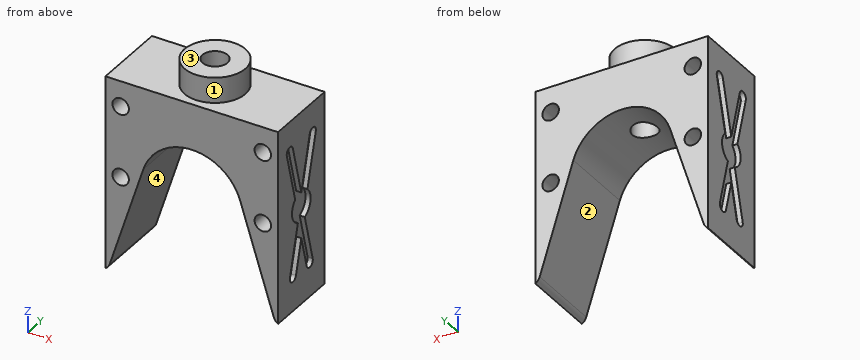
Autodesk Inventor part; units mm, degrees
ref_plane "Work Plane1" through (-17, 0, 0) normal (1, 0, 0) x (0, 1, 0)
ref_plane "XZ Plane" through (0, 0, 0) normal (0, 1, 0) x (-1, 0, 0)
ref_plane "XY Plane" through (0, 0, 0) normal (0, 0, 1) x (1, 0, 0)
sketch "Sketch1" plane through (0, 0, 0) normal (0, 1, 0) x (-1, 0, 0)
  line L0 (0, 0) -> (34, 0)
  line L1 (34, 0) -> (34, -38)
  line L2 (34, -38) -> (0, -38)
  line L3 (0, -38) -> (0, 0)
  point P0 (17, -38)
  dimension "d0" = 34
  dimension "d1" = 38
extrude "Extrusion1" add sketch "Sketch1" along normal blind 15
sketch "Sketch2" plane through (0, 15, 0) normal (0, 1, 0) x (1, 0, 0)
  arc A0 (-26.5342, 15.9835) -> (-7.4658, 15.9835) centre (-17, 19) ccw
  line L0 (-26.5342, 15.9835) -> (-33.5, 38)
  line L1 (0, 38) -> (-34, 38)
  line L2 (-7.4658, 15.9835) -> (-0.5, 38)
  point P0 (0, 0)
  point P1 (-17, 38)
  dimension "d4" = 16.5
  dimension "d5" = 16.5
  dimension "d6" = 10
  dimension "d7" = 19
extrude "Extrusion2" cut sketch "Sketch2" against normal up to surface (15 mm away)
fillet "Fillet1" radius 2 2 edges at (-0.5, 7.5, -38) (-33.5, 7.5, -38)
sketch "Sketch3" plane through (0, 15, 0) normal (0, 1, 0) x (1, 0, 0)
  line L0 (-34, 0) -> (0, 0)
  point P0 (-3, 19)
  point P1 (-31, 19)
  point P2 (-17, 0)
  point P3 (-17, 0)
  point P4 (-34, 38)
  dimension "d19" = 14
  dimension "d20" = 14
  dimension "d59" = 19
hole "Hole1" at (-3, 15, -19) at (-31, 15, -19) direction (0, -1, 0) diameter 3.242 depth 15
sketch "Sketch4" plane through (0, 15, 0) normal (0, 1, 0) x (1, 0, 0)
  line L0 (-34, 0) -> (0, 0)
  point P0 (-31, 5)
  point P1 (-3, 5)
  point P2 (-17, 0)
  point P3 (-17, 0)
  dimension "d28" = 14
  dimension "d29" = 14
  dimension "d30" = 5
hole "Hole2" at (-31, 15, -5) at (-3, 15, -5) direction (0, -1, 0) diameter 3.242 depth 15
sketch "Sketch5" plane through (-34, 0, 0) normal (0, 0, 1) x (1, 0, 0)
  circle A0 centre (17, 7.5) radius 6
  line L0 (0, 0) -> (34, 0)
  line L1 (0, 0) -> (0, 15)
  point P0 (17, 0)
  point P1 (0, 7.5)
  dimension "d31" = 12
extrude "Extrusion3" add sketch "Sketch5" along normal blind 5
sketch "Sketch6" plane through (-17, 7.5, 5) normal (0, 0, 1) x (1, 0, 0)
  circle A0 centre (0, 0) radius 6
  point P0 (17, -7.5)
hole "Hole3" at (-17, 7.5, 5) direction (0, 0, -1) diameter 4.917 depth 15
sketch "Sketch7" plane through (-34, 0, -38) normal (-1, 0, 0) x (0, 0, 1)
  line L0 (16.5986, 8.6063) -> (7.046, 11.1659)
  arc A0 (7.046, 11.1659) -> (6.5283, 9.2341) centre (6.7872, 10.2) ccw
  line L1 (6.5283, 9.2341) -> (13, 7.5)
  line L2 (13, 7.5) -> (6.5283, 5.7659)
  arc A1 (6.5283, 5.7659) -> (7.046, 3.8341) centre (6.7872, 4.8) ccw
  line L3 (7.046, 3.8341) -> (16.5986, 6.3937)
  line L4 (21.653, 9.4662) -> (31.7283, 12.1659)
  arc A2 (32.246, 10.2341) -> (31.7283, 12.1659) centre (31.9872, 11.2) ccw
  line L5 (32.246, 10.2341) -> (22.0423, 7.5)
  line L6 (22.0423, 7.5) -> (32.246, 4.7659)
  arc A3 (31.7283, 2.8341) -> (32.246, 4.7659) centre (31.9872, 3.8) ccw
  line L7 (31.7283, 2.8341) -> (21.653, 5.5338)
  line L8 (0, 0) -> (0, 15)
  line L9 (0, 7.5) -> (36.5337, 7.5) construction
  arc A4 (16.5986, 6.3937) -> (21.653, 5.5338) centre (19.3872, 7.5) ccw
  arc A5 (21.653, 9.4662) -> (16.5986, 8.6063) centre (19.3872, 7.5) ccw
  line L10 (0, 15) -> (38, 15)
  point P0 (38, 0)
  point P1 (11.8223, 5.1139)
  dimension "d42" = 2
  dimension "d43" = 2
  dimension "d44" = 2
  dimension "d45" = 2
  dimension "d46" = 12.6
  dimension "d47" = 12.6
  dimension "d48" = 26
  dimension "d49" = 26
  dimension "d50" = 30
  dimension "d51" = 30
  dimension "d52" = 3.8
  dimension "d53" = 3
  dimension "d54" = 3
  dimension "d55" = 13
extrude "Extrusion4" cut sketch "Sketch7" against normal blind 1
ref_plane "Work Plane1" through (-17, 0, 0) normal (1, 0, 0) x (0, 1, 0)
mirror "Mirror1" about plane through (-17, 0, 0) normal (1, 0, 0) of "Extrusion4"
equation "\"d5\" = d4"
equation "\"d12\" = d20"
equation "\"d44\" = d43"
equation "\"d47\" = d46"
equation "\"d54\" = d53"
properties part number "2023"
The listing builds one solid part. Answer for the finished solid, in the listing's coordinates (mm). Face numbers are marked on the shaded views. Coordinates: 2 decimals unless noted, no trailing zeros. Write each loop counter-clockwise with the first axis right and the second up, starting at its lowest first coordinate (ties: lowest second). Pieces come first, ordered by that corner, then holes. Notation, with made-up numbers: M 55,84.5 L 59,84.5 A30 ccw 59,115.5 Z; hole C -11.5,-22 d8. An arc over 180 degrees is marked long. Use a Markdown table: item, result. Add a question column.
1. Section B-B (z = -2) is taken. Give the vertices of the cut face in (x, y).
2. Section D-D (z = -19) is taken. Give the vertices of the cut face in (x, y).
3. Given P1, Ø1.9, axis at x = -31, z = -5, coming from the +Y side, flat-ended and moving along its own axis, determine where the tip first touches the part or whether it passes through.
4. Straight lines are drawn through the part: line 1 along X through (y, z) = (5.5, -5); line 2 along X through (y, z) = (7.5, -5); line 3 along X through (y, z) = (11.5, -11). For each, find the intervals that lie inside material, in ascending order. Write a range as [from, to].
5. Section C-C (x = -3) is taken. Give the vertices of the cut face in (y, z), plus the area to 3 significant figures.
6. Section A-A (x = -17) is taken. Give the vertices of the cut face in (y, z), plus the area to 3 significant figures.
7. For a pull along X with two mould halves and no side action, classify the marked faces 1, 2, 3 and 4 as +X half, -X half, draft (parallel to the pull), parting line (faces both ways), or undercut.
Data:
| question | item | result |
|---|---|---|
| 1 | outline | M -34,0 L 0,0 L 0,15 L -34,15 Z; hole C -17,7.5 d4.92 |
| 2 | outline | M -34,0 L -32.62,0 L -32.62,15 L -34,15 L -34,10.47 L -33,10.47 L -33,4.53 L -34,4.53 Z; M -29.38,0 L -27.49,0 L -27.49,15 L -29.38,15 Z; M -6.51,0 L -4.62,0 L -4.62,15 L -6.51,15 Z; M -1.38,0 L 0,0 L 0,4.53 L -1,4.53 L -1,10.47 L 0,10.47 L 0,15 L -1.38,15 Z |
| 3 | P1 | passes through |
| 4 | line 1 | x = [-34, -32.62], [-29.38, -18.43], [-15.57, -4.62], [-1.38, 0] |
| 4 | line 2 | x = [-34, -32.62], [-29.38, -19.46], [-14.54, -4.62], [-1.38, 0] |
| 4 | line 3 | x = [-34, -23], [-11, 0] |
| 5 | outline | M 0,-30.1 L 15,-30.1 L 15,-20.62 L 0,-20.62 Z; M 0,-17.38 L 15,-17.38 L 15,-6.62 L 0,-6.62 Z; M 0,-3.38 L 15,-3.38 L 15,0 L 0,0 Z |
| 5 | area | 354 mm2 |
| 6 | outline | M 0,-9 L 5.04,-9 L 5.04,5 L 1.5,5 L 1.5,0 L 0,0 Z; M 9.96,-9 L 15,-9 L 15,0 L 13.5,0 L 13.5,5 L 9.96,5 Z |
| 6 | area | 126 mm2 |
| 7 | face 1 | parting line |
| 7 | face 2 | undercut |
| 7 | face 3 | draft |
| 7 | face 4 | undercut |
